The listing builds one solid part. Answer for the finished solid, in the listing's coordinates (mm). Coordinates: 2 decimals unless noted, no trailing zeros. Write each loop counter-clockwise with the first axis right and the second up, starting at its lowest first coordinate (ties: lowest second). Pieces come first, ordered by that corner, then holes. Notation, with made-up numbers: M 28.25,24.5 L 38.25,24.5 A10 cw 38.25,30.5 Z; hole C 25.25,-39.75 d1. An arc over 180 degrees is marked long. Put each result on its own line as item: value. Start each with the question number.
```python
from build123d import *

# Parameters (mm, degrees)
BOSS_EXTRUDE1_DEPTH = 19.05
SKETCH2_W           = 43.434
SKETCH2_H           = 13.97
MOTOR_HOLE_DEPTH    = 19.05
SKETCH3_W           = 6.35
SKETCH3_H           = 12.7
CUT_EXTRUDE2_DEPTH  = 36.941
SKETCH5_W           = 6.35
SKETCH5_H           = 13.97
SKETCH5_H_2         = 6.35
CUT_EXTRUDE6_DEPTH  = 36.941
SKETCH7_W           = 45.976326486
SKETCH7_H           = 159.787423729
CUT_EXTRUDE7_DEPTH  = 20.05


with BuildPart() as part:
    # Sketch1 → Boss-Extrude1 (new body)
    with BuildSketch(Plane(origin=(0, 0, 0), x_dir=(1, 0, 0), z_dir=(0, 1, 0))):
        Polygon((-10.033, 66.167), (-11.6205, 66.167), (-11.6205, 76.835), (-17.9705, 76.835), (-17.9705, -78.867), (-11.6205, -78.867), (-11.6205, -66.167), (11.6205, -66.167), (11.6205, -78.867), (17.9705, -78.867), (17.9705, 76.835), (11.6205, 76.835), (11.6205, 66.167), (10.033, 66.167), (10.033, 59.817), (11.6205, 59.817), (11.6205, -59.817), (-11.6205, -59.817), (-11.6205, 59.817), (-10.033, 59.817), align=None)
    extrude(amount=BOSS_EXTRUDE1_DEPTH)

    # Sketch2 → Motor Hole (cut)
    with BuildSketch(Plane.ZY.offset(17.9705)):
        with Locations((29.972, 12.065)):
            Rectangle(SKETCH2_W, SKETCH2_H)
    extrude(amount=-MOTOR_HOLE_DEPTH, mode=Mode.SUBTRACT)

    # Sketch3 → Cut-Extrude2 (cut, through all)
    with BuildSketch(Plane.ZY.offset(17.9705)):
        with Locations((-73.66, 6.35)):
            Rectangle(SKETCH3_W, SKETCH3_H)
    extrude(amount=-CUT_EXTRUDE2_DEPTH, mode=Mode.SUBTRACT)

    # Sketch5 → Cut-Extrude6 (cut, through all)
    with BuildSketch(Plane.ZY.offset(17.9705)):
        with Locations((62.992, 12.065)):
            Rectangle(SKETCH5_W, SKETCH5_H)
        with Locations((-62.992, 9.525)):
            Rectangle(SKETCH5_W, SKETCH5_H_2)
    extrude(amount=-CUT_EXTRUDE6_DEPTH, mode=Mode.SUBTRACT)

    # Sketch7 → Cut-Extrude7 (cut, through all)
    with BuildSketch(Plane(origin=(0, 0, 0), x_dir=(1, 0, 0), z_dir=(0, 1, 0))):
        with Locations((-11.367663243, 1.026711865)):
            Rectangle(SKETCH7_W, SKETCH7_H)
    extrude(amount=CUT_EXTRUDE7_DEPTH, mode=Mode.SUBTRACT)


solid = part.part
```
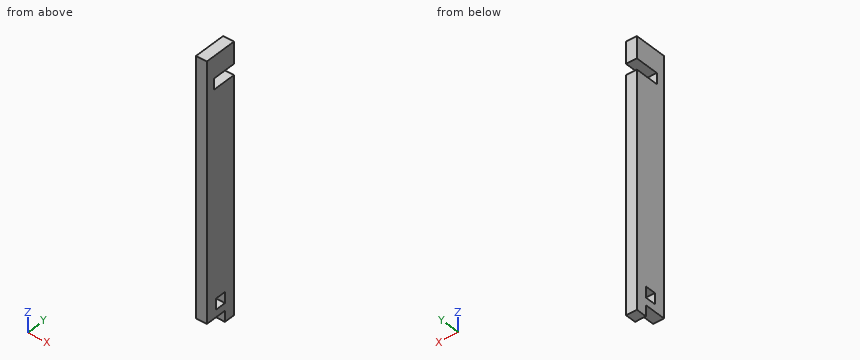
1) Given pin 1 Ø1.9 at (x, y) = (15.5, 10.5) entering from -Z (3 decimals); pin 2 Ø3 at (x, z) = (13, -72.5) entering from -Y, each flat-ended and moving along its own axis, determine where each tip first touches the part or whether it passes through.
2) A cutting plane is placed at C-C on y = 14.25. Write down the section's boundary in (x, z) (1 decimal), then the cut area to 3 significant figures.
3) A cutting plane is placed at A-A on y = 8.5. Write down the section's boundary in (x, z) (1 decimal), then the cut area to 3 significant figures.
4) A cutting plane is placed at B-B on x = 16. Write down the section's boundary in (y, z) (3 decimals), then the cut area to 3 significant figures.
5) Straight lines are drawn through the part: probe 1 along Z at (x, y) = (12, 8) (3 decimals); probe 2 along Z at (x, y) = (17.5, 18.25) (3 decimals); probe 3 along Y at (x, z) = (13.75, -63). For each, find the intervals that lie inside material, in ascending order.
6) A cutting plane is placed at D-D on z = -64. Write down the section's boundary in (x, y).
Answers follow:
1. pin 1: stops at z = -70.485
1. pin 2: stops at y = 12.7
2. outline: M 11.6,-76.8 L 18,-76.8 L 18,59.8 L 11.6,59.8 Z; M 11.6,66.2 L 18,66.2 L 18,78.9 L 11.6,78.9 Z
2. area: 948 mm²
3. outline: M 11.6,-70.5 L 18,-70.5 L 18,-66.2 L 11.6,-66.2 Z; M 11.6,-59.8 L 18,-59.8 L 18,59.8 L 11.6,59.8 Z; M 11.6,66.2 L 18,66.2 L 18,78.9 L 11.6,78.9 Z
3. area: 868 mm²
4. outline: M 0,-70.485 L 12.7,-70.485 L 12.7,-76.835 L 19.05,-76.835 L 19.05,59.817 L 5.08,59.817 L 5.08,66.167 L 19.05,66.167 L 19.05,78.867 L 0,78.867 Z; hole M 6.35,-66.167 L 12.7,-66.167 L 12.7,-59.817 L 6.35,-59.817 Z
4. area: 2,760 mm²
5. probe 1: z = -70.485 to -66.167, -59.817 to 59.817, 66.167 to 78.867
5. probe 2: z = -76.835 to 59.817, 66.167 to 78.867
5. probe 3: y = 0 to 6.35, 12.7 to 19.05
6. outline: M 11.62,0 L 17.97,0 L 17.97,6.35 L 11.62,6.35 Z; M 11.62,12.7 L 17.97,12.7 L 17.97,19.05 L 11.62,19.05 Z
